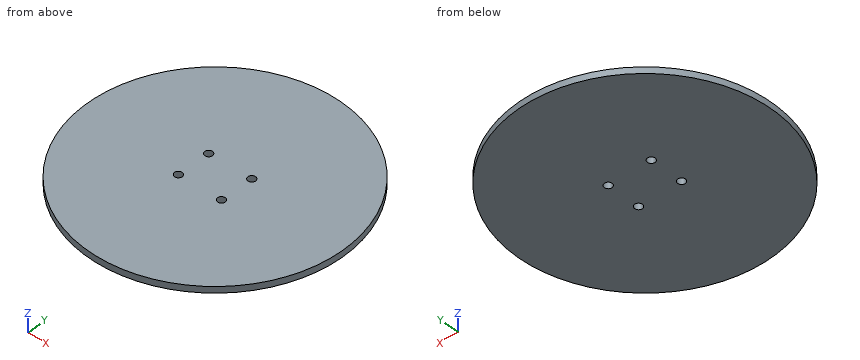
```python
from build123d import *

# Parameters (mm, degrees)
F0_R     = 50
F0_R_2   = 1.5
F1_DEPTH = 2.5


with BuildPart() as f1:
    # F0 (on Top) → F1 (new body)
    with BuildSketch(Plane.XY):
        Circle(F0_R)
        with Locations((-8.5, -6.5)):
            Circle(F0_R_2, mode=Mode.SUBTRACT)
        with Locations((8.5, -6.5)):
            Circle(F0_R_2, mode=Mode.SUBTRACT)
        with Locations((-8.5, 6.5)):
            Circle(F0_R_2, mode=Mode.SUBTRACT)
        with Locations((8.5, 6.5)):
            Circle(F0_R_2, mode=Mode.SUBTRACT)
    extrude(amount=-F1_DEPTH)


solid = f1.part
```
Geometry check sheet. Reference: the model listing, model coordinates, mm. Give positions to 0.01 mm unless a question says otherwise; leave off trailing zeros. Order: outer loops, then holes, each group sorted by start corner. A loop starts at its lowest first (then second) coordinate and runs counter-clockwise, first axis right, second up. Notation, with made-up numbers: (43, 42) -> (76, 42) arc R11 ccw to (76, 51) -> close; hole circle Ø3 at (66, -30). An arc over 180 degrees is marked (long way). Write each question's results on one line, items separated by ' | '. Start each with the question number.
(1) Sectioned sample at D-D (y = -26). Enter the section's corners in (x, z), plus the area to 3 significant figures.
(2) Sectioned sample at C-C (y = -6.5). Enter the section's corners in (x, z).
(3) Scan lines: line 1 (Y direction, x = 8.5, z = -1.25); line 2 (X direction, y = 7.5, z = -0.8); line 3 (Y direction, x = -1.5, z = -2.35). Record each from-to range of solid material in increasing order.
(4) Sectioned sample at A-A (x = -8.5). Enter the section's corners in (y, z), plus the area to 3 significant figures.
(5) Gauge pin test, flat ends, axial feed: P1, Ø1, axis at x = -10.5, z = -1, coming from the -Y side; P2, Ø1.5, axis at y = -17.5, z = -2, coming from the +X side; P3, Ø1, axis at y = -7, z = -2, coming from the -X side. Record the tip position at first contact, or that the pin passes through.
(6) Sectioned sample at B-B (z = -2). Enter the section's corners in (x, y).
Answer below:
1) outline: (-42.71, -2.5) -> (42.71, -2.5) -> (42.71, 0) -> (-42.71, 0) -> close | area: 214 mm2
2) outline: (-49.58, -2.5) -> (-10, -2.5) -> (-10, 0) -> (-49.58, 0) -> close; (-7, -2.5) -> (7, -2.5) -> (7, 0) -> (-7, 0) -> close; (10, -2.5) -> (49.58, -2.5) -> (49.58, 0) -> (10, 0) -> close
3) line 1: -49.27 to -8, -5 to 5, 8 to 49.27 | line 2: -49.43 to -9.62, -7.38 to 7.38, 9.62 to 49.43 | line 3: -49.98 to 49.98
4) outline: (-49.27, -2.5) -> (-8, -2.5) -> (-8, 0) -> (-49.27, 0) -> close; (-5, -2.5) -> (5, -2.5) -> (5, 0) -> (-5, 0) -> close; (8, -2.5) -> (49.27, -2.5) -> (49.27, 0) -> (8, 0) -> close | area: 231 mm2
5) P1: y = -48.99 | P2: x = 47.11 | P3: x = -49.58
6) outline: circle Ø100 at (0, 0); hole circle Ø3 at (-8.5, -6.5); hole circle Ø3 at (-8.5, 6.5); hole circle Ø3 at (8.5, -6.5); hole circle Ø3 at (8.5, 6.5)
